CAD build for the part. Positions are in the model's coordinates, mm. A direction names the side the tool comes from. Round coordinates to 2 decimals unless told otherwise and drop trailing zeros. Loops run counter-clockwise (first coordinate to the right, second up) from the corner with the lowest first, then second, coordinate; pieces in that order, holes last.
from build123d import *

# Parameters (mm, degrees)
SKETCH1_W             = 98.679
SKETCH1_H             = 73.2282
BOSS_EXTRUDE1_DEPTH   = 3.175
SKETCH2_W             = 83.2866
SKETCH2_H             = 54.7878
BOSS_EXTRUDE2_DEPTH   = 9.525
F_4_CLEARANCE_HOLE1_D = 3.2639


with BuildPart() as part:
    # Sketch1 → Boss-Extrude1 (new body)
    with BuildSketch(Plane.XY):
        Rectangle(SKETCH1_W, SKETCH1_H)
    extrude(amount=BOSS_EXTRUDE1_DEPTH)

    # Sketch2 → Boss-Extrude2 (add)
    with BuildSketch(Plane.XY.offset(3.175)):
        Rectangle(SKETCH2_W, SKETCH2_H)
    extrude(amount=BOSS_EXTRUDE2_DEPTH)

    # #4 Clearance Hole1 (through all)
    with Locations(Plane(origin=(-44.3357, 31.7373, 12.7), x_dir=(1, 0, 0), z_dir=(0, 0, 1))):
        with Locations((0, 0), (88.6714, 0), (88.6714, -63.4746), (0, -63.4746)):
            Hole(F_4_CLEARANCE_HOLE1_D / 2)


solid = part.part
Item 1: Wall check: L1, parallel to Y at x = 7.5, z = 10.5; L2, parallel to X at y = -1, z = 7.25; L3, parallel to Z at x = 31.5, y = -31 (3 decimals). Give the ranges that are in metal, low to high.
Verdict:
L1: y = -27.39 to 27.39
L2: x = -41.64 to 41.64
L3: z = 0 to 3.175
Item 2: Flat gauge pins, fed straight in: P1, Ø5, axis at y = -1.5, z = 8.5, coming from the +X side; P2, Ø7.5, axis at x = 13.5, z = 6.5, coming from the -Y side; P3, Ø2, axis at x = -44.34, y = 31.74, coming from the -Z side; P4, Ø5, axis at x = -36.5, z = 10, coming from the -Y side. Where does each tip first touch, or does it go through?
Verdict:
P1: stops at x = 41.64
P2: stops at y = -36.61
P3: passes through
P4: stops at y = -27.39
Item 3: Mould opens along Y. For faces 1 (the flat face through (0, 30, 3.175)), 2 (the cylindrical face through (-45.9, 32.2, 1.6)), 3 (the flat face through (-1, 27.394, 8)) say: released by +Y, released by -Y, zero draft, split by the parting line, or undercut.
Verdict:
face 1: zero draft
face 2: undercut
face 3: released by +Y
Item 4: Cut at B-B (x = -5). List the corners of the cut face in (y, z) (3 decimals), plus the area to 3 significant figures.
Verdict:
outline: (-36.614, 0) - (36.614, 0) - (36.614, 3.175) - (27.394, 3.175) - (27.394, 12.7) - (-27.394, 12.7) - (-27.394, 3.175) - (-36.614, 3.175) - close
area: 754 mm2
Item 5: Cut at D-D (y = 29). List the corners of the cut face in (x, z) (1 decimal), plus the area to 3 significant figures.
Verdict:
outline: (-49.3, 0) - (49.3, 0) - (49.3, 3.2) - (-49.3, 3.2) - close
area: 313 mm2
Item 6: Cut at C-C (z = 6.25). List the corners of the cut face in (x, y), plus the area to 3 significant figures.
Verdict:
outline: (-41.64, -27.39) - (41.64, -27.39) - (41.64, 27.39) - (-41.64, 27.39) - close
area: 4,560 mm2
Item 7: 3-axis set-ups, long thin cutter, end or side, ignore diameter. For faces 4 (the flat face through (41.643, 0, 8)), 5 (the flat face through (-41.643, 0, 8)), 6 (the flat face through (-1, -27.394, 8)): which of +Z, -Z, +X, -X, +Y, -Y reach the whole face in a straight line?
Verdict:
face 4: +Z, +X, +Y, -Y
face 5: +Z, -X, +Y, -Y
face 6: +Z, +X, -X, -Y
Item 8: Cut at A-A (y = 6.5). List the corners of the cut face in (x, z) (1 decimal), plus the area to 3 significant figures.
Verdict:
outline: (-49.3, 0) - (49.3, 0) - (49.3, 3.2) - (41.6, 3.2) - (41.6, 12.7) - (-41.6, 12.7) - (-41.6, 3.2) - (-49.3, 3.2) - close
area: 1,110 mm2
